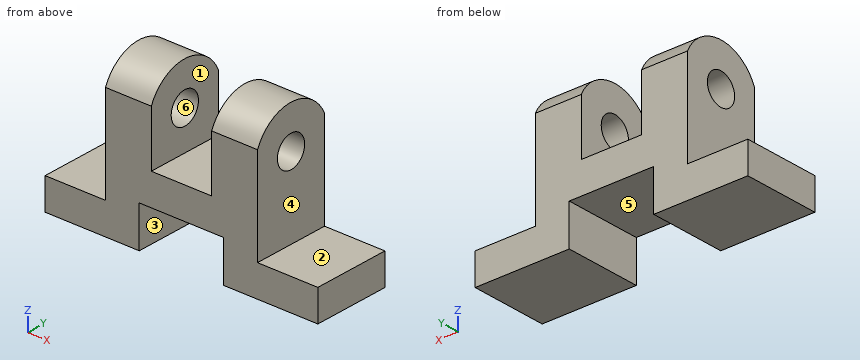
from build123d import *

# Parameters (mm, degrees)
F0_W     = 113
F0_H     = 64
F1_DEPTH = 32
F2_R     = 6.5
F3_DEPTH = 113.001
F4_W     = 35
F4_H     = 17
F4_W_2   = 25
F4_H_2   = 51
F4_H_3   = 34
F5_DEPTH = 32.001


with BuildPart() as f1:
    # F0 (on Front) → F1 (new body)
    with BuildSketch(Plane.XZ):
        with Locations((0, 32)):
            Rectangle(F0_W, F0_H)
    extrude(amount=-F1_DEPTH)

    # F2 (on face) → F3 (cut, through all)
    with BuildSketch(Plane.YZ.offset(56.5)):
        with Locations((16, 46)):
            Circle(F2_R)
        with BuildLine():
            Line((0, 64), (0, 53.088723))
            ThreePointArc((0, 53.088723), (16, 63.5), (32, 53.088723))
            Line((32, 53.088723), (32, 64))
            Line((32, 64), (0, 64))
        make_face()
    extrude(amount=-F3_DEPTH, mode=Mode.SUBTRACT)

    # F4 (on Front) → F5 (cut, through all)
    with BuildSketch(Plane.XZ):
        with Locations((0, 8.5)):
            Rectangle(F4_W, F4_H)
        with Locations((-44, 38.5)):
            Rectangle(F4_W_2, F4_H_2)
        with Locations((44, 38.5)):
            Rectangle(F4_W_2, F4_H_2)
        with Locations((0, 47)):
            Rectangle(F4_W_2, F4_H_3)
    extrude(amount=-F5_DEPTH, mode=Mode.SUBTRACT)


solid = f1.part
Read the model definition and answer for the solid it produces. Units are mm, in the model's axes. Face numbers are marked on the shaded views. A direction names the side the tool comes from. Give positions to 0.01 mm unless a question says otherwise; leave off trailing zeros. Write each loop counter-clockwise with the first axis right and the second up, starting at its lowest first coordinate (ties: lowest second). Pieces come first, ordered by that corner, then holes. Notation, with made-up numbers: M 39,-4 L 70,-4 A28 cw 70,21 Z; hole C 62,-0.5 d5. An arc over 180 degrees is marked long. One line per item, written item: value. Start each with the question number.
(1) Flat-ended cylindrical pins translate along their axes: pin 1 Ø9.5 at (y, z) = (15, 27) entering from -X; pin 2 Ø4 at (x, y) = (42.5, 28.5) entering from +Z; pin 3 Ø1 at (y, z) = (8, 24.5) entering from +X; pin 4 Ø11.5 at (y, z) = (16, 46) entering from +X. Find the tip coordinate at first contact, or state that the pin passes through.
(2) Find section C-C (z = 46). Determine the outline of the cut face in (x, y).
(3) Find section D-D (y = 5.5). Determine the outline of the cut face in (x, z).
(4) Find section A-A (y = 16). Determine the outline of the cut face in (x, z), plus the area to 3 significant figures.
(5) A tool of negligible diameter and unlimited length cuts with its end or side. For the marked faces 1, 2 and 3, from which of +Z, -Z, +X, -X, +Y, -Y can it reach the whole face along a straight path? Write none if from no direction.
(6) Find the intervals of material crossed by line 1 (X direction, y = 30, z = 41); line 2 (Z direction, x = -23.5, y = 16); line 3 (X direction, y = 23, z = 27), in increasing order.
(7) Determine the mould class of the marked faces 4, 5 and 6 for opening direction Z: pulls with the +Z half, pulls with the -Z half, needs draft (parallel to the pull), parting line crosses it, or undercut.
(8) Find section B-B (z = 33). Determine the outline of the cut face in (x, y).
Results below:
1. pin 1: stops at x = -31.5
1. pin 2: stops at z = 13
1. pin 3: stops at x = 31.5
1. pin 4: passes through
2. outline: M -31.5,0 L -12.5,0 L -12.5,9.5 L -31.5,9.5 Z; M -31.5,22.5 L -12.5,22.5 L -12.5,32 L -31.5,32 Z; M 12.5,0 L 31.5,0 L 31.5,9.5 L 12.5,9.5 Z; M 12.5,22.5 L 31.5,22.5 L 31.5,32 L 12.5,32 Z
3. outline: M -56.5,0 L -17.5,0 L -17.5,17 L 17.5,17 L 17.5,0 L 56.5,0 L 56.5,13 L 31.5,13 L 31.5,60 L 12.5,60 L 12.5,30 L -12.5,30 L -12.5,60 L -31.5,60 L -31.5,13 L -56.5,13 Z
4. outline: M -56.5,0 L -17.5,0 L -17.5,17 L 17.5,17 L 17.5,0 L 56.5,0 L 56.5,13 L 31.5,13 L 31.5,39.5 L 12.5,39.5 L 12.5,30 L -12.5,30 L -12.5,39.5 L -31.5,39.5 L -31.5,13 L -56.5,13 Z; M -31.5,52.5 L -12.5,52.5 L -12.5,63.5 L -31.5,63.5 Z; M 12.5,52.5 L 31.5,52.5 L 31.5,63.5 L 12.5,63.5 Z
4. area: 2,720 mm^2
5. face 1: +Z, +Y, -Y
5. face 2: +Z, +X, +Y, -Y
5. face 3: -Z, +Y, -Y
6. line 1: x = -31.5 to -12.5, 12.5 to 31.5
6. line 2: z = 0 to 39.5, 52.5 to 63.5
6. line 3: x = -31.5 to 31.5
7. face 4: needs draft
7. face 5: pulls with the -Z half
7. face 6: undercut
8. outline: M -31.5,0 L -12.5,0 L -12.5,32 L -31.5,32 Z; M 12.5,0 L 31.5,0 L 31.5,32 L 12.5,32 Z
